```python
from build123d import *

# Parameters (mm, degrees)
SKETCH_1_W      = 5.25
SKETCH_1_H      = 2.5
EXTRUDE_1_DEPTH = 1.42
SKETCH_2_R      = 0.725
EXTRUDE_2_DEPTH = 5
SKETCH_3_R      = 0.965
EXTRUDE_3_DEPTH = 0.5


with BuildPart() as part:
    # ｽｹｯﾁ1 → ﾎﾞｽ - 押し出し1 (new body)
    with BuildSketch(Plane.XY):
        Rectangle(SKETCH_1_W, SKETCH_1_H)
    extrude(amount=EXTRUDE_1_DEPTH)

    # ｽｹｯﾁ2 → ﾎﾞｽ - 押し出し2 (add)
    with BuildSketch(Plane(origin=(0, 0, 0), x_dir=(-1, 0, 0), z_dir=(0, 0, -1))):
        with Locations(Location((-1.27, 0, 0), (0, 0, 180))):
            Circle(SKETCH_2_R)
        with Locations(Location((1.27, 0, 0), (0, 0, 180))):
            Circle(SKETCH_2_R)
    extrude(amount=EXTRUDE_2_DEPTH)

    # ｽｹｯﾁ3 → ﾎﾞｽ - 押し出し3 (add)
    with BuildSketch(Plane.XY.offset(1.42)):
        with Locations((-1.27, 0)):
            Circle(SKETCH_3_R)
        with Locations((1.27, 0)):
            Circle(SKETCH_3_R)
    extrude(amount=EXTRUDE_3_DEPTH)


solid = part.part
```
Source: CAD feature listing. Evaluate the final solid. Frame: model axes, mm. A direction names the side the tool comes from. Give positions to 0.01 mm unless a question says otherwise; leave off trailing zeros. Loops run counter-clockwise (first coordinate to the right, second up) from the corner with the lowest first, then second, coordinate; pieces in that order, holes last. Notation, with made-up numbers: (-25.75, 17) -> (-12.75, 17) arc R24 cw to (-12.75, 41) -> close; hole circle Ø5 at (16, -17). An arc over 180 degrees is marked (long way). Put each result on its own line as item: value. Start each with the question number.
1) Contact query for flat-ended pins moving along their axis: P1, Ø1.5, axis at x = -2, z = -3.5, coming from the +Y side (3 decimals); P2, Ø1.5, axis at x = -1.5, y = 1, coming from the -Z side. Output: stop coordinate, or through.
2) Cut plane D-D (y = -0.5). Return loops of the section in (x, z) (3 decimals).
3) Cut plane A-A (y = 0). Return loops of the section in (x, z) (3 decimals), then the cut area to 3 significant figures.
4) Cut plane B-B (x = 1.27). Return loops of the section in (y, z) (3 decimals), then the cut area to 3 significant figures.
5) Draft query along X for faces 1 (the face through (1.96, -0.22, -2.46)), 2 (the face through (-2.625, 0, 1)), 3 (the face through (0, -1.25, 1)), 4 (the face through (2.625, 0, 1)). Return one class per face: released by +X, released by -X, zero draft, split by the parting line, or undercut.
6) Reachability of faces 5 (the face through (-1.845, 0.441, -2.465)), 6 (the face through (0, 0, 1.42)), 7 (the face through (1, 0, -5)) from +Z, -Z, +X, -X, +Y, -Y: full face, straight path, thin tool, end or side. Return the list, or none.
7) Cut plane C-C (z = -4.25). Return loops of the section in (x, y) (3 decimals), then the cut area to 3 significant figures.
8) Material intervals for probe 1 along Z at (x, y) = (-0.3, -0.6); probe 2 along X at (y, z) = (0.45, -1); probe 3 along X at (y, z) = (0.35, -0.5), sorted ascending.
Results are:
1. P1: stops at y = 0.725
1. P2: stops at z = -5
2. outline: (-2.625, 0) -> (-1.795, 0) -> (-1.795, -5) -> (-0.745, -5) -> (-0.745, 0) -> (0.745, 0) -> (0.745, -5) -> (1.795, -5) -> (1.795, 0) -> (2.625, 0) -> (2.625, 1.42) -> (2.095, 1.42) -> (2.095, 1.92) -> (0.445, 1.92) -> (0.445, 1.42) -> (-0.445, 1.42) -> (-0.445, 1.92) -> (-2.095, 1.92) -> (-2.095, 1.42) -> (-2.625, 1.42) -> close
3. outline: (-2.625, 0) -> (-1.995, 0) -> (-1.995, -5) -> (-0.545, -5) -> (-0.545, 0) -> (0.545, 0) -> (0.545, -5) -> (1.995, -5) -> (1.995, 0) -> (2.625, 0) -> (2.625, 1.42) -> (2.235, 1.42) -> (2.235, 1.92) -> (0.305, 1.92) -> (0.305, 1.42) -> (-0.305, 1.42) -> (-0.305, 1.92) -> (-2.235, 1.92) -> (-2.235, 1.42) -> (-2.625, 1.42) -> close
3. area: 23.9 mm2
4. outline: (-1.25, 0) -> (-0.725, 0) -> (-0.725, -5) -> (0.725, -5) -> (0.725, 0) -> (1.25, 0) -> (1.25, 1.42) -> (0.965, 1.42) -> (0.965, 1.92) -> (-0.965, 1.92) -> (-0.965, 1.42) -> (-1.25, 1.42) -> close
4. area: 11.8 mm2
5. face 1: undercut
5. face 2: released by -X
5. face 3: zero draft
5. face 4: released by +X
6. face 5: -Z
6. face 6: +Z
6. face 7: -Z, +X, -X, +Y, -Y
7. outline: circle Ø1.45 at (-1.27, 0); circle Ø1.45 at (1.27, 0)
7. area: 3.30 mm2
8. probe 1: z = 0 to 1.42
8. probe 2: x = -1.84 to -0.7, 0.7 to 1.84
8. probe 3: x = -1.9 to -0.64, 0.64 to 1.9
